from build123d import *

# Parameters (mm, degrees)
SKETCH_1_W          = 49
SKETCH_1_H          = 40
EXTRUDE_1_DEPTH     = 3
SKETCH_2_R          = 1.55
SKETCH_2_R_2        = 7
CUT_EXTRUDE_1_DEPTH = 36.131894341
CUT_EXTRUDE_2_DEPTH = 36.131894341
FILLET_1_R          = 2


with BuildPart() as part:
    # 草图1 → 凸台-拉伸1 (new body)
    with BuildSketch(Plane(origin=(0, 0, 0), x_dir=(1, 0, 0), z_dir=(0, 1, 0))):
        with Locations((0, 5)):
            Rectangle(SKETCH_1_W, SKETCH_1_H)
        with BuildLine():
            Line((-19, 21.6), (-18.5, 21.6))
            ThreePointArc((-18.5, 21.6), (-16.9, 20), (-18.5, 18.4))
            Line((-18.5, 18.4), (-19, 18.4))
            ThreePointArc((-19, 18.4), (-20.6, 20), (-19, 21.6))
        make_face(mode=Mode.SUBTRACT)
        with BuildLine():
            Line((19, 18.4), (18.5, 18.4))
            ThreePointArc((18.5, 18.4), (16.9, 20), (18.5, 21.6))
            Line((18.5, 21.6), (19, 21.6))
            ThreePointArc((19, 21.6), (20.6, 20), (19, 18.4))
        make_face(mode=Mode.SUBTRACT)
        with BuildLine():
            Line((19, 1.6), (18.5, 1.6))
            ThreePointArc((18.5, 1.6), (16.9, 0), (18.5, -1.6))
            Line((18.5, -1.6), (19, -1.6))
            ThreePointArc((19, -1.6), (20.6, 0), (19, 1.6))
        make_face(mode=Mode.SUBTRACT)
        with BuildLine():
            Line((-19, -1.6), (-18.5, -1.6))
            ThreePointArc((-18.5, -1.6), (-16.9, 0), (-18.5, 1.6))
            Line((-18.5, 1.6), (-19, 1.6))
            ThreePointArc((-19, 1.6), (-20.6, 0), (-19, -1.6))
        make_face(mode=Mode.SUBTRACT)
    extrude(amount=EXTRUDE_1_DEPTH)

    # 草图2 → 切除-拉伸1 (cut, through all)
    with BuildSketch(Plane(origin=(0, 3, 0), x_dir=(1, 0, 0), z_dir=(0, 1, 0))):
        with Locations(Location((9.192388155, 14.192388155, 0), (0, 0, 270))):
            Circle(SKETCH_2_R)
        with Locations(Location((9.192388155, -4.192388155, 0), (0, 0, 90))):
            Circle(SKETCH_2_R)
        with Locations(Location((-9.192388155, 14.192388155, 0), (0, 0, 90))):
            Circle(SKETCH_2_R)
        with Locations(Location((-9.192388155, -4.192388155, 0), (0, 0, 270))):
            Circle(SKETCH_2_R)
        with Locations(Location((0, 5, 0), (0, 0, 270))):
            Circle(SKETCH_2_R_2)
    extrude(amount=-CUT_EXTRUDE_1_DEPTH, mode=Mode.SUBTRACT)

    # 草图3 → 切除-拉伸2 (cut, through all)
    with BuildSketch(Plane(origin=(0, 3, 0), x_dir=(1, 0, 0), z_dir=(0, 1, 0))):
        Polygon((-15.721322439, 25), (-11.036685955, 19.411212236), (11.036685955, 19.411212236), (15.721322439, 25), align=None)
        Polygon((15.721322439, -15), (11.036685955, -9.411212236), (-11.036685955, -9.411212236), (-15.721322439, -15), align=None)
    extrude(amount=-CUT_EXTRUDE_2_DEPTH, mode=Mode.SUBTRACT)

    # 圆角1
    fillet_1_edges = [part.edges().sort_by_distance(p)[0] for p in [
        (-15.721322439, 1.5, -25),
        (15.721322439, 1.5, -25),
        (11.036685955, 1.5, -19.411212236),
        (-11.036685955, 1.5, -19.411212236),
        (15.721322439, 1.5, 15),
        (-15.721322439, 1.5, 15),
        (-11.036685955, 1.5, 9.411212236),
        (11.036685955, 1.5, 9.411212236),
        (24.5, 1.5, 15),
        (-24.5, 1.5, 15),
        (-24.5, 1.5, -25),
        (24.5, 1.5, -25),
    ]]
    fillet(fillet_1_edges, radius=FILLET_1_R)


solid = part.part
Here's how the part is built. I have some questions about the finished solid (model axes, mm). A direction names the side the tool comes from. Coordinates: 2 decimals unless noted, no trailing zeros. Order: outer loops, then holes, each group sorted by start corner. A loop starts at its lowest first (then second) coordinate and runs counter-clockwise, first axis right, second up.
Item 1: If we section it at C-C on z = 0: List the corners of the cut face in (x, y) for me, plus the area to 3 significant figures.
Result sheet:
outline: (-24.5, 0) - (-20.6, 0) - (-20.6, 3) - (-24.5, 3) - close; (-16.9, 0) - (-4.9, 0) - (-4.9, 3) - (-16.9, 3) - close; (4.9, 0) - (16.9, 0) - (16.9, 3) - (4.9, 3) - close; (20.6, 0) - (24.5, 0) - (24.5, 3) - (20.6, 3) - close
area: 95.4 mm2
Item 2: If we mould it in two halves opening along Z, with no side actions, what happens to faces 5 (the face through (13.4, 1.52, 12.23)), 6 (the face through (-16.9, 1.5, 0)), 7 (the face through (-13.4, 1.52, -22.23)), 8 (the face through (-10.136, 1.521, 2.962))? For each: +Z half, -Z half, draft (parallel to the pull), parting line (faces both ways), or undercut.
Result sheet:
face 5: +Z half
face 6: undercut
face 7: -Z half
face 8: undercut
Item 3: For faces 1 (the face through (-23.93, 1.52, 14.4)), 2 (the face through (13.355, 1.521, -22.176)), 3 (the face through (16.9, 1.5, -20)), 4 (the face through (15.82, 1.479, 14.818)), which set-ups out of +Z, -Z, +X, -X, +Y, -Y let a thin tool reach every point of the face, with its end or its side?
Result sheet:
face 1: +Z, -X, +Y, -Y
face 2: -Z, +Y, -Y
face 3: +Y, -Y
face 4: +Z, +Y, -Y
Item 4: I need wall thicknesses on line 1 (X direction, y = 1.1, z = 4); line 2 (Z direction, x = -10, y = 2.4); line 3 (Z direction, x = 8, y = 0.85). Which ranges of each line are inside material? Lowest first, please.
Result sheet:
line 1: x = -24.5 to -10.73, -7.65 to 7.65, 10.73 to 24.5
line 2: z = -19.41 to -15.52, -12.87 to 2.87, 5.52 to 9.41
line 3: z = -19.41 to -15.18, -13.2 to 3.2, 5.18 to 9.41
Item 5: For P1, Ø1.9, axis at x = 9.19, z = 4.19, coming from the +Y side, with a flat end and sliding along its axis, tell me the tip position at first contact or that it passes through.
Result sheet:
P1: passes through
Item 6: If we section it at D-D on y = 0.95: State how many separate pieces and enclosed holes the cut face has, plus the area to 3 significant figures.
Result sheet:
separate pieces: 1
enclosed holes: 9
area: 1,430 mm2
Item 7: If we section it at A-A on z = -5: List the corners of the cut face in (x, y) for me, plus the area to 3 significant figures.
Result sheet:
outline: (-24.5, 0) - (-7, 0) - (-7, 3) - (-24.5, 3) - close; (7, 0) - (24.5, 0) - (24.5, 3) - (7, 3) - close
area: 105 mm2
Item 8: If we section it at B-B on x = -1: List the corners of the cut face in (y, z) for me.
Result sheet:
outline: (0, -19.41) - (3, -19.41) - (3, -11.93) - (0, -11.93) - close; (0, 1.93) - (3, 1.93) - (3, 9.41) - (0, 9.41) - close
